The listing builds one solid part. Answer for the finished solid, in the listing's coordinates (mm). A direction names the side the tool comes from. Coordinates: 2 decimals unless noted, no trailing zeros. Loops run counter-clockwise (first coordinate to the right, second up) from the corner with the lowest first, then second, coordinate; pieces in that order, holes last. Notation, with made-up numbers: (79.25, 51.5) - (86.25, 51.5) arc R15 cw to (86.25, 64.5) - close; hole circle Ø8 at (75.5, -8). An arc over 180 degrees is marked (long way). Use one line per item in the form item = value. Start each with the question number.
```python
from build123d import *

# Parameters (mm, degrees)
SKETCH1_W                      = 64
SKETCH1_H                      = 14.75
BASE_FLANGE1_DEPTH             = 1.5
EDGE_FLANGE1_STRIP_W           = 9.3
EDGE_FLANGE1_STRIP_H           = 1.5
EDGE_FLANGE1_STRIP_CUT_DEPTH   = 14.75
EDGE_FLANGE1_STRIP_2_W         = 9.3
EDGE_FLANGE1_STRIP_2_H         = 1.5
EDGE_FLANGE1_STRIP_CUT_2_DEPTH = 14.75
EDGE_FLANGE1_DEPTH             = 14.75
EDGE_FLANGE1_BEND_DEPTH        = 14.75
FILLET1_R                      = 6


# Sheet-metal steps are written as plain solids
with BuildPart() as part:
    # Sketch1 → Base-Flange1 (new body)
    with BuildSketch(Plane(origin=(0, 0, 0), x_dir=(1, 0, 0), z_dir=(0, 1, 0))):
        with Locations((32, 7.375)):
            Rectangle(SKETCH1_W, SKETCH1_H)
    extrude(amount=-BASE_FLANGE1_DEPTH)

    # Edge-Flange1 strip (across the edge) → Edge-Flange1 strip cut (cut)
    with BuildSketch(Plane(origin=(0, -1.5, 0), x_dir=(1, 0, 0), z_dir=(0, 0, -1))):
        with Locations((-1.5, -0.75)):
            Rectangle(EDGE_FLANGE1_STRIP_W, EDGE_FLANGE1_STRIP_H)
    extrude(amount=EDGE_FLANGE1_STRIP_CUT_DEPTH, mode=Mode.SUBTRACT)

    # Edge-Flange1 strip 2 (across the edge) → Edge-Flange1 strip cut 2 (cut)
    with BuildSketch(Plane(origin=(64, -1.5, -14.75), x_dir=(-1, 0, 0), z_dir=(0, 0, 1))):
        with Locations((-1.5, -0.75)):
            Rectangle(EDGE_FLANGE1_STRIP_2_W, EDGE_FLANGE1_STRIP_2_H)
    extrude(amount=EDGE_FLANGE1_STRIP_CUT_2_DEPTH, mode=Mode.SUBTRACT)

    # Edge-Flange1 section (across the edge) → Edge-Flange1 (add)
    with BuildSketch(Plane(origin=(0, -1.5, 0), x_dir=(1, 0, 0), z_dir=(0, 0, -1))):
        with BuildLine():
            Line((0, 1.65), (0, 7))
            Line((0, 7), (1.5, 7))
            Line((1.5, 7), (1.5, 1.65))
            ThreePointArc((1.5, 1.65), (1.983273811, 0.483273811), (3.15, 0))
            Line((3.15, 0), (3.15, -1.5))
            ThreePointArc((3.15, -1.5), (0.922613639, -0.577386361), (0, 1.65))
        make_face()
    extrude(amount=EDGE_FLANGE1_DEPTH)

    # Edge-Flange1 section 2 (across the edge) → Edge-Flange1 bend (add)
    with BuildSketch(Plane(origin=(64, -1.5, -14.75), x_dir=(-1, 0, 0), z_dir=(0, 0, 1))):
        with BuildLine():
            Line((0, 1.65), (0, 7))
            Line((0, 7), (1.5, 7))
            Line((1.5, 7), (1.5, 1.65))
            ThreePointArc((1.5, 1.65), (1.983273811, 0.483273811), (3.15, 0))
            Line((3.15, 0), (3.15, -1.5))
            ThreePointArc((3.15, -1.5), (0.922613639, -0.577386361), (0, 1.65))
        make_face()
    extrude(amount=EDGE_FLANGE1_BEND_DEPTH)

    # Fillet1
    fillet1_edges = [part.edges().sort_by_distance(p)[0] for p in [
        (0.75, -8.5, 0),
        (63.25, -8.5, 0),
    ]]
    fillet(fillet1_edges, radius=FILLET1_R)


solid = part.part
```
(1) A cutting plane is placed at D-D (y = -7). Determine the outline of the cut face in (x, z), then the cut area to 3 significant figures.
(2) A cutting plane is placed at C-C (x = 35.5). Determine the outline of the cut face in (y, z), then the cut area to 3 significant figures.
(3) Find the intervals of material crossed by probe 1 along X at (y, z) = (-7, -8.5); probe 2 along X at (y, z) = (-2.5, -14); probe 3 along Y at (x, z) = (32, -13.75), in increasing order. Write a range as from..to.
(4) This flat-tipped pin is pushed along its axis until it touches: pin 1 Ø3 at (x, z) = (9.5, -9) entering from -Y. Where does it stop, or does it pass through?
(5) A cutting plane is placed at B-B (y = -4). Determine the outline of the cut face in (x, z).
(6) For faces 1 (the face through (0.828, -6.696, -1.711)), 2 (the face through (1.5, -6, -7)), determine the directions among +Z, -Z, +X, -X, +Y, -Y from which every point of the face is accessible in a straight line to the end or side of a thin tool.
(7) A cutting plane is placed at A-A (z = -8.25). Determine the outline of the cut face in (x, y).
(8) Determine the mould class of faces 3 (the face through (62.5, -6, -7)), 4 (the face through (64, -6, -7)), 5 (the face through (32, 0, -7)), 6 (the face through (1.971, -1.996, -7.272)) for opening direction X: +X half, -X half, draft (parallel to the pull), parting line (faces both ways), or undercut.
Evaluation:
q1.outline = (0, -14.75) - (1.5, -14.75) - (1.5, -2.03) - (0, -2.03) - close; (62.5, -14.75) - (64, -14.75) - (64, -2.03) - (62.5, -2.03) - close
q1.area = 38.2 mm^2
q2.outline = (-1.5, -14.75) - (0, -14.75) - (0, 0) - (-1.5, 0) - close
q2.area = 22.1 mm^2
q3.probe_1 = 0..1.5, 62.5..64
q3.probe_2 = 0.07..1.63, 62.37..63.93
q3.probe_3 = -1.5..0
q4.pin_1 = -1.5
q5.outline = (0, -14.75) - (1.5, -14.75) - (1.5, -0.19) - (0, -0.19) - close; (62.5, -14.75) - (64, -14.75) - (64, -0.19) - (62.5, -0.19) - close
q6.face_1 = +Z, +X, -X, -Y
q6.face_2 = +Z, -Z, -Y
q7.outline = (0, -8.5) - (1.5, -8.5) - (1.5, -3.15) arc R1.65 cw to (3.15, -1.5) - (60.85, -1.5) arc R1.65 cw to (62.5, -3.15) - (62.5, -8.5) - (64, -8.5) - (64, -3.15) arc R3.15 ccw to (60.85, 0) - (3.15, 0) arc R3.15 ccw to (0, -3.15) - close
q8.face_3 = undercut
q8.face_4 = +X half
q8.face_5 = draft
q8.face_6 = undercut
